from build123d import *

# Parameters (mm, degrees)
F0_W     = 1
F0_H     = 11
F1_DEPTH = 25
F3_DEPTH = 50
F4_R     = 2.6
F5_DEPTH = 41.001
F6_SIZE  = 1


with BuildPart() as f1:
    # F0 (on Front) → F1 (new body, symmetric)
    with BuildSketch(Plane.XZ):
        with Locations((26.5, 15.5)):
            Rectangle(F0_W, F0_H)
        with Locations((-26.5, 15.5)):
            Rectangle(F0_W, F0_H)
        Polygon((9.3024417906, -20), (14.6689019081, -14), (-14.6689019081, -14), (-9.3024417906, -20), align=None)
        Polygon((26, 10), (26, 9), (27, 10), align=None)
        Polygon((-27, 10), (-26, 9), (-26, 10), align=None)
        with BuildLine():
            ThreePointArc((4.3588989435, 9), (8.4731632061, 5.310885546), (10, 0))
            ThreePointArc((10, 0), (-5.310885546, -8.4731632061), (-4.3588989435, 9))
            Line((-4.3588989435, 9), (-26, 9))
            Line((-26, 9), (-26, -14))
            Line((-26, -14), (-14.6689019081, -14))
            Line((-14.6689019081, -14), (14.6689019081, -14))
            Line((14.6689019081, -14), (26, -14))
            Line((26, -14), (26, 9))
            Line((26, 9), (4.3588989435, 9))
        make_face()
        with BuildLine():
            Line((-26, 9), (-4.3588989435, 9))
            ThreePointArc((-4.3588989435, 9), (-2.2360679957, 9.7467943406), (-3.73e-08, 10))
            Line((-3.73e-08, 10), (-26, 10))
            Line((-26, 10), (-26, 9))
        make_face()
        Polygon((-26, 10), (-3.73e-08, 10), (26, 10), (26, 21), (-26, 21), align=None)
        with BuildLine():
            ThreePointArc((-3.73e-08, 10), (2.2360679593, 9.746794349), (4.3588989435, 9))
            Line((4.3588989435, 9), (26, 9))
            Line((26, 9), (26, 10))
            Line((26, 10), (-3.73e-08, 10))
        make_face()
    extrude(amount=F1_DEPTH, both=True)

    # F2 (on Front) → F3 (cut, symmetric)
    with BuildSketch(Plane.XZ):
        Polygon((11.6050554439, 20), (12.4383887773, 21), (-12.4383887773, 21), (-11.6050554439, 20), align=None)
    extrude(amount=F3_DEPTH, both=True, mode=Mode.SUBTRACT)

    # F4 (on face) → F5 (cut, through all)
    with BuildSketch(Plane.XY.offset(21)):
        with Locations((20, 20)):
            Circle(F4_R)
        with Locations((-20, 20)):
            Circle(F4_R)
        with Locations((-20, -20)):
            Circle(F4_R)
        with Locations((20, -20)):
            Circle(F4_R)
    extrude(amount=-F5_DEPTH, mode=Mode.SUBTRACT)

    # F6
    f6_edges = [f1.edges().sort_by_distance(p)[0] for p in [
        (17.4, -20, 21),
        (-22.6, -20, 21),
        (-22.6, 20, 21),
        (17.4, 20, 21),
        (17.4, 20, -14),
        (-22.6, 20, -14),
        (17.4, -20, -14),
        (-22.6, -20, -14),
    ]]
    chamfer(f6_edges, length=F6_SIZE)


solid = f1.part
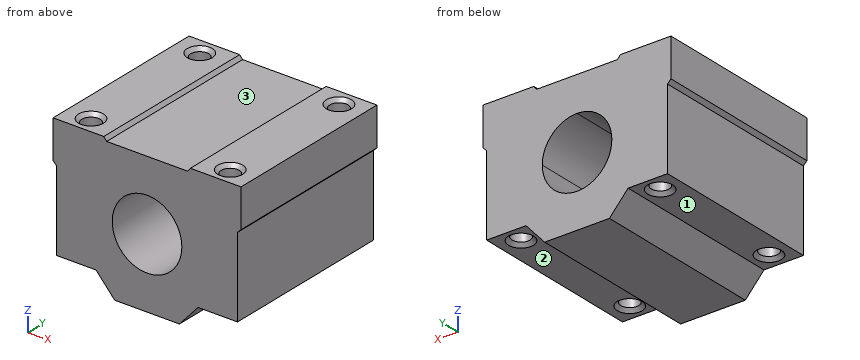
Work out the finished part from the listing and answer in its coordinate system (mm). Face numbers are marked on the shaded views. A direction names the side the tool comes from. Round coordinates to 2 decimals unless told otherwise and drop trailing zeros. Loops run counter-clockwise (first coordinate to the right, second up) from the corner with the lowest first, then second, coordinate; pieces in that order, holes last. Notation, with made-up numbers: (-26.5, 71.5) -> (28.5, 71.5) arc R17 ccw to (28.5, 100.5) -> close; hole circle Ø8 at (14.5, -37). An arc over 180 degrees is marked (long way). Use one line per item in the form item = value.
(1) A tool of negligible diameter and unlimited length cuts with its end or side. For the marked faces 1, 2 and 3, from which of +Z, -Z, +X, -X, +Y, -Y can it reach the whole face along a straight path? Write none if from no direction.
Answer list:
face_1 = -Z, -X, +Y, -Y
face_2 = -Z, +X, +Y, -Y
face_3 = +Z, +Y, -Y
(2) Find section D-D on y = 5.5. Give the vertices of the cut face in (x, z).
Answer list:
outline = (-27, 10) -> (-26, 9) -> (-26, -14) -> (-14.67, -14) -> (-9.3, -20) -> (9.3, -20) -> (14.67, -14) -> (26, -14) -> (26, 9) -> (27, 10) -> (27, 21) -> (12.44, 21) -> (11.61, 20) -> (-11.61, 20) -> (-12.44, 21) -> (-27, 21) -> close; hole circle Ø20 at (0, 0)
(3) Flat-ended cylindrical pins translate along their axes: P1, Ø7, axis at x = -20, y = -20, coming from the +Z side; P2, Ø12, axis at y = 8.5, z = -5.5, coming from the +X side; P3, Ø9, axis at x = 20.5, y = 7.5, coming from the -Z side; P4, Ø3, axis at x = 20, y = -20, coming from the -Z side. Find the tip coordinate at first contact, or state that the pin passes through.
Answer list:
P1 = 20.9
P2 = 26
P3 = -14
P4 = through
(4) Find section C-C on z = -7. Give the vertices of the cut face in (x, y).
Answer list:
outline = (-26, -25) -> (-7.14, -25) -> (-7.14, 25) -> (-26, 25) -> close; (7.14, -25) -> (26, -25) -> (26, 25) -> (7.14, 25) -> close; hole circle Ø5.2 at (-20, -20); hole circle Ø5.2 at (-20, 20); hole circle Ø5.2 at (20, -20); hole circle Ø5.2 at (20, 20)
(5) Straight lines are drawn through the part: line 1 (Y direction, x = 20, z = 2); line 2 (X direction, y = 21, z = -13.5); line 3 (Z direction, x = 0, y = -2). For each, find the intervals that lie inside material, in ascending order.
Answer list:
line_1 = -25 to -22.6, -17.4 to 17.4, 22.6 to 25
line_2 = -26 to -22.93, -17.07 to 17.07, 22.93 to 26
line_3 = -20 to -10, 10 to 20
(6) Find section A-A on y = 20. Give the number of separate pieces and of enclosed holes in the cut face, then the cut area to 3 significant figures.
Answer list:
separate_pieces = 3
enclosed_holes = 1
area = 1,280 mm2
(7) Find section B-B on x = 20. Give the vertices of the cut face in (y, z).
Answer list:
outline = (-25, -14) -> (-23.6, -14) -> (-22.6, -13) -> (-22.6, 20) -> (-23.6, 21) -> (-25, 21) -> close; (-17.4, -13) -> (-16.4, -14) -> (16.4, -14) -> (17.4, -13) -> (17.4, 20) -> (16.4, 21) -> (-16.4, 21) -> (-17.4, 20) -> close; (22.6, -13) -> (23.6, -14) -> (25, -14) -> (25, 21) -> (23.6, 21) -> (22.6, 20) -> close
